from build123d import *

# Parameters (mm, degrees)
SKETCH1_W           = 42
SKETCH1_H           = 57
SKETCH1_R           = 1.6
SKETCH1_R_2         = 11.25
BOSS_EXTRUDE1_DEPTH = 3
FILLET1_R           = 5


with BuildPart() as part:
    # Sketch1 → Boss-Extrude1 (new body)
    with BuildSketch(Plane(origin=(0, 0, 0), x_dir=(1, 0, 0), z_dir=(0, 1, 0))):
        with Locations((21, 28.5)):
            Rectangle(SKETCH1_W, SKETCH1_H)
        with Locations((36.5, 51.5)):
            Circle(SKETCH1_R, mode=Mode.SUBTRACT)
        with Locations((5.5, 51.5)):
            Circle(SKETCH1_R, mode=Mode.SUBTRACT)
        with Locations((5.5, 20.5)):
            Circle(SKETCH1_R, mode=Mode.SUBTRACT)
        with Locations((36.5, 20.5)):
            Circle(SKETCH1_R, mode=Mode.SUBTRACT)
        with Locations((6, 7.5)):
            Circle(SKETCH1_R, mode=Mode.SUBTRACT)
        with Locations((36, 7.5)):
            Circle(SKETCH1_R, mode=Mode.SUBTRACT)
        with Locations((21, 36)):
            Circle(SKETCH1_R_2, mode=Mode.SUBTRACT)
    extrude(amount=BOSS_EXTRUDE1_DEPTH)

    # Fillet1
    fillet1_edges = [part.edges().sort_by_distance(p)[0] for p in [
        (0, 1.5, -57),
        (42, 1.5, -57),
        (42, 1.5, 0),
        (0, 1.5, 0),
    ]]
    fillet(fillet1_edges, radius=FILLET1_R)


solid = part.part
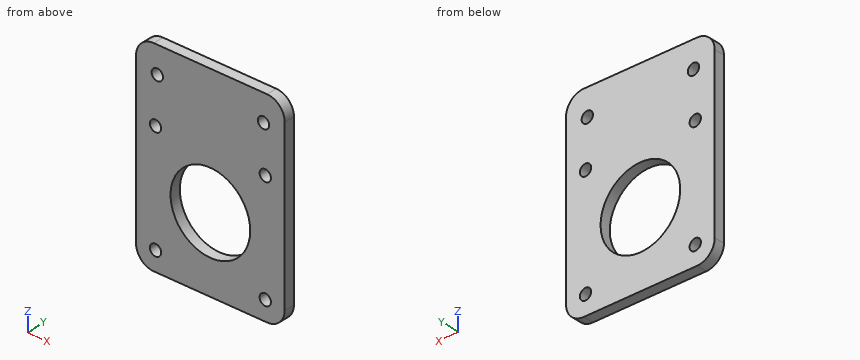
Geometry: final body of the model. Coordinates: model frame, mm. Coordinates: 2 decimals unless noted, no trailing zeros. Loops run counter-clockwise (first coordinate to the right, second up) from the corner with the lowest first, then second, coordinate; pieces in that order, holes last. Notation, with made-up numbers: (52, 88) - (72, 88) arc R13 ccw to (72, 98) - close; hole circle Ø6 at (46.25, 88.5). An arc over 180 degrees is marked (long way). Put each result on its own line as item: value. Start each with the question number.
Q1. Cut plane D-D, the plane z = -32.5. Return loops of the section in (x, y), and give its area (3 significant figures).
Q2. Cut plane A-A, the plane z = -20.5. Return loops of the section in (x, y), and give its area (3 significant figures).
Q3. Pin query (flat end, axial travel): pin 1 Ø5 at (x, z) = (36.5, -51.5) entering from -Y. Return the tip coordinate at first contact, or that it passes through.
Q4. Cut plane C-C, the plane y = 1.7. Return loops of the section in (x, z).
Q5. Cut plane B-B, the plane x = 13. Return loops of the section in (y, z).
Q6. Line query: line 1 (X direction, y = 1.9, z = -7.5); line 2 (Z direction, x = 36.5, y = 1.6); line 3 (Z direction, x = 6, y = 2.75). Output: solid intervals per line, ascending.
Filled sheet:
1. outline: (0, 0) - (10.31, 0) - (10.31, 3) - (0, 3) - close; (31.69, 0) - (42, 0) - (42, 3) - (31.69, 3) - close
1. area: 61.8 mm²
2. outline: (0, 0) - (3.9, 0) - (3.9, 3) - (0, 3) - close; (7.1, 0) - (34.9, 0) - (34.9, 3) - (7.1, 3) - close; (38.1, 0) - (42, 0) - (42, 3) - (38.1, 3) - close
2. area: 107 mm²
3. pin 1: y = 0
4. outline: (0, -52) arc R5 ccw to (5, -57) - (37, -57) arc R5 ccw to (42, -52) - (42, -5) arc R5 ccw to (37, 0) - (5, 0) arc R5 ccw to (0, -5) - close; hole circle Ø3.2 at (5.5, -51.5); hole circle Ø3.2 at (5.5, -20.5); hole circle Ø3.2 at (6, -7.5); hole circle Ø22.5 at (21, -36); hole circle Ø3.2 at (36, -7.5); hole circle Ø3.2 at (36.5, -51.5); hole circle Ø3.2 at (36.5, -20.5)
5. outline: (0, -57) - (3, -57) - (3, -43.91) - (0, -43.91) - close; (0, -28.09) - (3, -28.09) - (3, 0) - (0, 0) - close
6. line 1: 0 to 4.4, 7.6 to 34.4, 37.6 to 42
6. line 2: -57 to -53.1, -49.9 to -22.1, -18.9 to -9.02, -5.98 to 0
6. line 3: -57 to -53.02, -49.98 to -22.02, -18.98 to -9.1, -5.9 to 0
